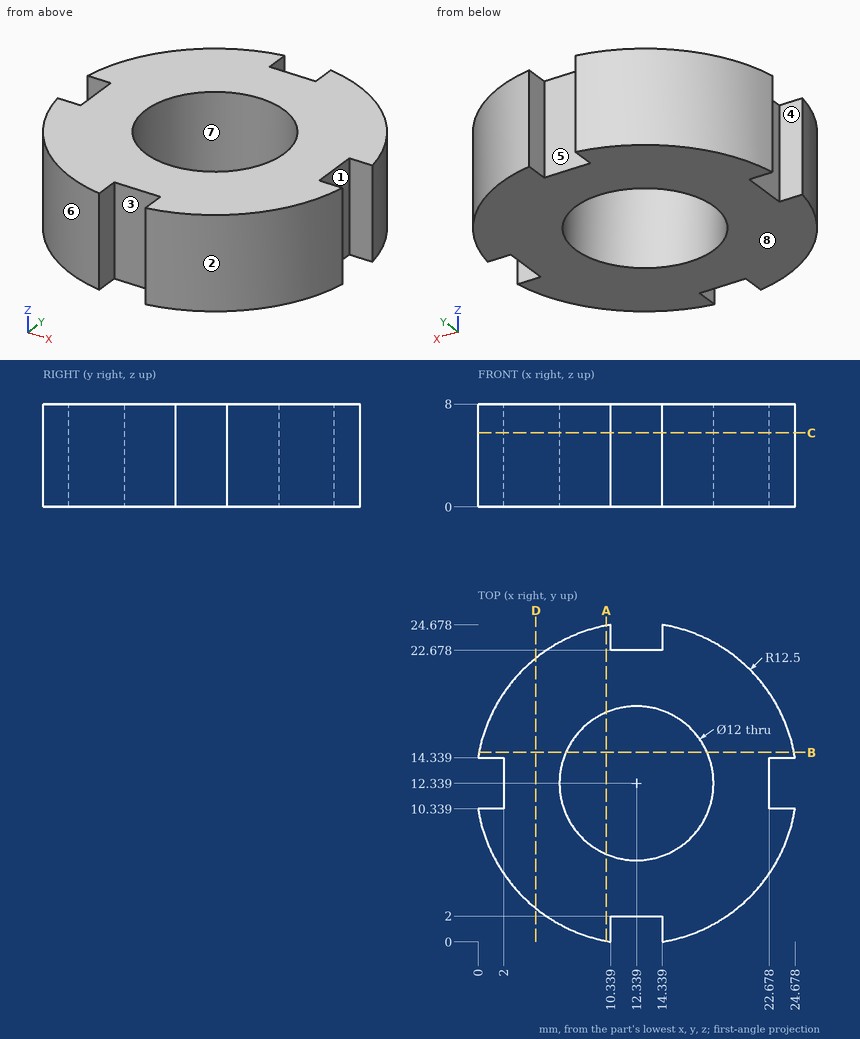
Study the drawing (mm; zero at the part's minimum x, y, z) and answer. A direction names the side the tool comes from. Round coordinates to 2 decimals unless told otherwise and drop trailing zeros. Order: outer loops, then holes, each group sorted by start corner. A loop starts at its lowest first (then second) coordinate and runs counter-clockwise, first axis right, second up. Notation, with made-up numbers: (-18.75, 62) - (10.25, 62) arc R19 ccw to (10.25, 67) - close; hole circle Ø3 at (-29, -38). An arc over 180 degrees is marked (long way). Use one line per item in the form item = value. Start each with the question number.
(1) The part is cut by section B-B (y = 14.75). Give the vertices of the cut face in (x, z), then the cut area to 3 significant figures.
(2) The part is cut by section C-C (z = 5.75). Give the vertices of the cut face in (x, y), then the cut area to 3 significant figures.
(3) Find the intervals of material crossed by line 1 along Y through (x, z) = (12.5, 0.75); line 2 along Y through (x, z) = (1, 7.25); line 3 along X through (y, z) = (12, 3.5), in increasing order. Write a range as from..to.
(4) Flat-ended cylindrical pins translate along their axes: pin 1 Ø1.5 at (y, z) = (4, 3.5) entering from +X; pin 2 Ø3 at (y, z) = (12.5, 2.5) entering from +X; pin 3 Ø0.6 at (y, z) = (24, 3) entering from -X. Find the tip coordinate at first contact, or state that the pin passes through.
(5) Determine the mould class of the marked faces 6, 7 and 8 for opening direction X: +X half, -X half, draft (parallel to the pull), parting line (faces both ways), or undercut.
(6) The part is cut by section A-A (x = 10). Give the vertices of the cut face in (y, z).
(7) The part is cut by section D-D (x = 4.5). Give the vertices of the cut face in (y, z).
(8) For the marked faces 1, 2, 3, 4 and 5, determine the directions among +Z, -Z, +X, -X, +Y, -Y from which every point of the face is accessible in a straight line to the end or side of a thin tool.
Checked values:
q1.outline = (0.07, 0) - (6.84, 0) - (6.84, 8) - (0.07, 8) - close; (17.83, 0) - (24.6, 0) - (24.6, 8) - (17.83, 8) - close
q1.area = 108 mm^2
q2.outline = (0, 10.34) arc R12.5 ccw to (10.34, 0) - (10.34, 2) - (14.34, 2) - (14.34, 0) arc R12.5 ccw to (24.68, 10.34) - (22.68, 10.34) - (22.68, 14.34) - (24.68, 14.34) arc R12.5 ccw to (14.34, 24.68) - (14.34, 22.68) - (10.34, 22.68) - (10.34, 24.68) arc R12.5 ccw to (0, 14.34) - (2, 14.34) - (2, 10.34) - close; hole circle Ø12 at (12.34, 12.34)
q2.area = 344 mm^2
q3.line_1 = 2..6.34, 18.34..22.68
q3.line_2 = 7.08..10.34, 14.34..17.6
q3.line_3 = 2..6.35, 18.33..22.68
q4.pin_1 = 22.27
q4.pin_2 = 22.68
q4.pin_3 = 7.13
q5.face_6 = -X half
q5.face_7 = undercut
q5.face_8 = draft
q6.outline = (0.06, 0) - (6.81, 0) - (6.81, 8) - (0.06, 8) - close; (17.86, 0) - (24.62, 0) - (24.62, 8) - (17.86, 8) - close
q7.outline = (2.6, 0) - (22.08, 0) - (22.08, 8) - (2.6, 8) - close
q8.face_1 = +Z, -Z, +X
q8.face_2 = +Z, -Z, +X, -Y
q8.face_3 = +Z, -Z, -Y
q8.face_4 = +Z, -Z, -X
q8.face_5 = +Z, -Z, +Y
